Build history of the part. All positions in model axes, mm. Face numbers are marked on the shaded views. A direction names the side the tool comes from. Round coordinates to 2 decimals unless told otherwise and drop trailing zeros. Order: outer loops, then holes, each group sorted by start corner. A loop starts at its lowest first (then second) coordinate and runs counter-clockwise, first axis right, second up. Notation, with made-up numbers: M 78.25,81.5 L 119.25,81.5 A15 cw 119.25,104.5 Z; hole C 34.25,-33.5 d8. An arc over 180 degrees is marked long. One line per item, written item: value. Start each with the question number.
Item 1: Pin check, flat tips, straight feed: pin 1 (5 mm diameter, centred on x = 9, y = -2, fed in from +Z); pin 2 (2.5 mm diameter, centred on x = 0, z = -6.75, fed in from -Y); pin 3 (8 mm diameter, centred on x = -5, z = -13.5, fed in from -Y); pin 4 (10 mm diameter, centred on x = -2, y = -12.5, fed in from +Z). Stop position of each tip, or through.
Item 2: Band-saw the part on B-B, the plane z = 0. Write the cut outline in (x, y), then the cut area to 3 significant figures.
Item 3: Two-plate mould, pull along X, no slides. Class the marked faces 1, 2, 3 and 4: +X half, -X half, draft (parallel to the pull), parting line (faces both ways), or undercut.
Item 4: Probe L1, parallel to X at y = -21.55, z = -17.5; L2, parallel to X at y = 0.25, z = 0; L3, parallel to Y at x = 0, z = 10. List the from-to ranges inside material, lowest first.
Item 5: Tool access for the marked faces 5 and 6: list every direction of +Z, -Z, +X, -X, +Y, -Y with a clear straight run to the whole face (end or side of a thin tool).
Item 6: Band-saw the part on D-D, the plane x = 14.5. Write the cut outline in (y, z).
Item 7: Band-saw the part on C-C, the plane y = -9. Write the cut outline in (x, z), then the cut area to 3 significant figures.
Item 8: Band-saw the part on A-A, the plane x = 0. Write the cut outline in (y, z), then the cut area to 3 significant figures.
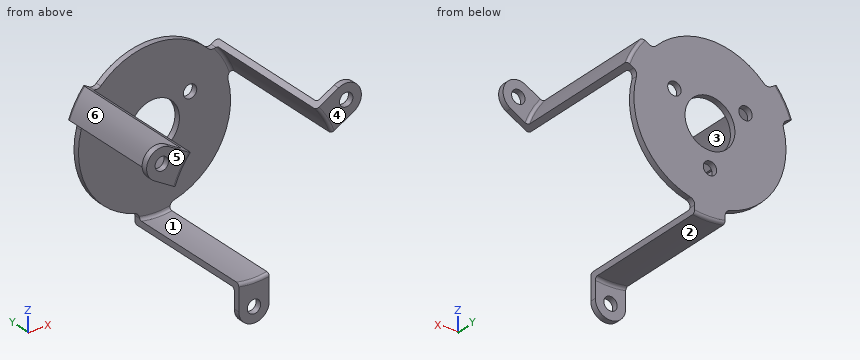
```python
from build123d import *

# Parameters (mm, degrees)
ESBO_O1_R                = 4.1
ESBO_O1_R_2              = 1.099999999999999
ESBO_O1_R_3              = 1.1000000000000312
ESBO_O1_R_4              = 1.1000000000000612
RESSALTO_EXTRUS_O1_DEPTH = 1
RESSALTO_EXTRUS_O2_START = 22.2
RESSALTO_EXTRUS_O2_DEPTH = 22.2
ESBO_O3_R                = 1.1
ESBO_O3_R_2              = 1.100000000000001
ESBO_O3_R_3              = 1.0999999999999976
RESSALTO_EXTRUS_O3_DEPTH = 1
FILETE1_R                = 1
FILETE2_R                = 0.5
FILETE3_R                = 0.5
FILETE4_R                = 0.5
FILETE5_R                = 0.5


with BuildPart() as part:
    # Esboço1 → Ressalto-extrusão1 (new body)
    with BuildSketch(Plane(origin=(0, 0, 0), x_dir=(1, 0, 0), z_dir=(0, 1, 0))):
        with BuildLine():
            Line((-2.5000000000000018, 14.2828568570857), (-2.5000000000000004, 12.24744871391589))
            ThreePointArc((-2.5000000000000004, 12.24744871391589), (-10.825317547305453, 6.250000000000052), (-11.856601717798243, -3.9586608474967395))
            Line((-11.856601717798243, -3.9586608474967395), (-13.619316876853024, -4.976364919081628))
            ThreePointArc((-13.619316876853024, -4.976364919081628), (-12.557368354874425, -7.249999999999881), (-11.119316876853064, -9.306491938003845))
            Line((-11.119316876853064, -9.306491938003845), (-9.356601717798284, -8.288787866418957))
            ThreePointArc((-9.356601717798284, -8.288787866418957), (-8.528e-14, -12.499999999999996), (9.356601717798178, -8.288787866419089))
            Line((9.356601717798178, -8.288787866419089), (11.119316876852942, -9.306491938004001))
            ThreePointArc((11.119316876852942, -9.306491938004001), (12.55736835487433, -7.250000000000061), (13.619316876852963, -4.976364919081819))
            Line((13.619316876852963, -4.976364919081819), (11.856601717798197, -3.958660847496907))
            ThreePointArc((11.856601717798197, -3.958660847496907), (10.8253175473055, 6.249999999999976), (2.499999999999998, 12.24744871391589))
            Line((2.499999999999998, 12.24744871391589), (2.4999999999999982, 14.2828568570857))
            ThreePointArc((2.4999999999999982, 14.2828568570857), (8.9e-16, 14.5), (-2.5000000000000018, 14.2828568570857))
        make_face()
        with Locations(Location((0, 0, 0), (0, 0, 270))):
            Circle(ESBO_O1_R, mode=Mode.SUBTRACT)
        with Locations(Location((0, 6.750000000000001, 0), (0, 0, 270))):
            Circle(ESBO_O1_R_2, mode=Mode.SUBTRACT)
        with Locations(Location((5.845671475544961, -3.374999999999999, 0), (0, 0, 270))):
            Circle(ESBO_O1_R_3, mode=Mode.SUBTRACT)
        with Locations(Location((-5.84567147554496, -3.3750000000000036, 0), (0, 0, 270))):
            Circle(ESBO_O1_R_4, mode=Mode.SUBTRACT)
    extrude(amount=RESSALTO_EXTRUS_O1_DEPTH)

    # Esboço2 → Ressalto-extrusão2 (add)
    with BuildSketch(Plane.XZ.offset(RESSALTO_EXTRUS_O2_START)):
        with BuildLine():
            Line((-11.11931687685307, 9.30649193800384), (-10.239125293076137, 8.798313090171801))
            ThreePointArc((-10.239125293076137, 8.798313090171801), (-11.691342951089984, 6.74999999999989), (-12.739125293076098, 4.4681860712495824))
            Line((-12.739125293076098, 4.4681860712495824), (-13.619316876853024, 4.976364919081628))
            ThreePointArc((-13.619316876853024, 4.976364919081628), (-12.557368354874427, 7.249999999999882), (-11.11931687685307, 9.30649193800384))
        make_face()
        with BuildLine():
            Line((-2.5000000000000018, -14.2828568570857), (-2.5000000000000013, -13.266499161421601))
            ThreePointArc((-2.5000000000000013, -13.266499161421601), (-2.17e-15, -13.500000000000002), (2.499999999999998, -13.266499161421601))
            Line((2.499999999999998, -13.266499161421601), (2.4999999999999982, -14.2828568570857))
            ThreePointArc((2.4999999999999982, -14.2828568570857), (8.9e-16, -14.500000000000002), (-2.5000000000000018, -14.2828568570857))
        make_face()
        with BuildLine():
            Line((13.619316876852963, 4.976364919081819), (12.739125293076041, 4.468186071249766))
            ThreePointArc((12.739125293076041, 4.468186071249766), (11.691342951089894, 6.750000000000058), (10.239125293076022, 8.798313090171948))
            Line((10.239125293076022, 8.798313090171948), (11.119316876852942, 9.306491938004001))
            ThreePointArc((11.119316876852942, 9.306491938004001), (12.557368354874331, 7.250000000000062), (13.619316876852963, 4.976364919081819))
        make_face()
    extrude(amount=-RESSALTO_EXTRUS_O2_DEPTH)

    # Esboço3 → Ressalto-extrusão3 (add)
    # profile 1 of 3: a face of its own
    with BuildSketch(Plane.XZ.offset(22.2)):
        with BuildLine():
            Line((2.4999999999999982, -14.2828568570857), (2.4999999999999982, -17.5))
            ThreePointArc((2.4999999999999982, -17.5), (-1.99e-15, -20), (-2.500000000000002, -17.5))
            Line((-2.500000000000002, -17.5), (-2.5000000000000018, -14.2828568570857))
            ThreePointArc((-2.5000000000000018, -14.2828568570857), (8.9e-16, -14.500000000000002), (2.4999999999999982, -14.2828568570857))
        make_face()
        with Locations(Location((-1.53e-15, -17.5, 0), (0, 0, 270))):
            Circle(ESBO_O3_R, mode=Mode.SUBTRACT)
    # profile 2 of 3: a face of its own
    with BuildSketch(Plane.XZ.offset(22.2)):
        with BuildLine():
            Line((-11.11931687685294, 9.306491938004003), (-13.905444566227628, 10.915063509461165))
            ThreePointArc((-13.905444566227628, 10.915063509461165), (-17.320508075688732, 10.000000000000085), (-16.40544456622765, 6.584936490538983))
            Line((-16.40544456622765, 6.584936490538983), (-13.619316876852961, 4.97636491908182))
            ThreePointArc((-13.619316876852961, 4.97636491908182), (-12.55736835487433, 7.250000000000063), (-11.11931687685294, 9.306491938004003))
        make_face()
        with Locations(Location((-15.15544456622764, 8.750000000000073, 0), (0, 0, 270))):
            Circle(ESBO_O3_R_2, mode=Mode.SUBTRACT)
    # profile 3 of 3: a face of its own
    with BuildSketch(Plane.XZ.offset(22.2)):
        with BuildLine():
            Line((13.619316876853029, 4.976364919081625), (16.40544456622774, 6.58493649053875))
            ThreePointArc((16.40544456622774, 6.58493649053875), (17.320508075688867, 9.999999999999838), (13.905444566227779, 10.915063509460968))
            Line((13.905444566227779, 10.915063509460968), (11.11931687685307, 9.306491938003841))
            ThreePointArc((11.11931687685307, 9.306491938003841), (12.557368354874429, 7.249999999999881), (13.619316876853029, 4.976364919081625))
        make_face()
        with Locations(Location((15.155444566227757, 8.749999999999858, 0), (0, 0, 270))):
            Circle(ESBO_O3_R_3, mode=Mode.SUBTRACT)
    extrude(amount=-RESSALTO_EXTRUS_O3_DEPTH)

    # Filete1
    filete1_edges = [part.edges().sort_by_distance(p)[0] for p in [
        (11.856601717798199, 0.5, 3.9586608474969074),
        (2.4999999999999982, 0.5, -12.24744871391589),
        (-2.5000000000000004, 0.5, -12.24744871391589),
        (-11.856601717798242, 0.5, 3.9586608474967386),
        (9.356601717798178, 0.5, 8.288787866419089),
        (-9.356601717798284, 0.5, 8.288787866418957),
    ]]
    fillet(filete1_edges, radius=FILETE1_R)

    # Filete2
    filete2_edges = [part.edges().sort_by_distance(p)[0] for p in [
        (-12.557368354874423, 1, 7.2499999999998845),
        (12.557368354874328, 1, 7.250000000000058),
        (-2.33e-15, 1, -14.5),
    ]]
    fillet(filete2_edges, radius=FILETE2_R)

    # Filete3
    filete3_edges = [part.edges().sort_by_distance(p)[0] for p in [
        (-1.67e-15, 0, -13.499999999999998),
        (11.691342951089894, 0, 6.750000000000058),
        (-11.691342951089982, 0, 6.749999999999892),
    ]]
    fillet(filete3_edges, radius=FILETE3_R)

    # Filete4
    filete4_edges = [part.edges().sort_by_distance(p)[0] for p in [
        (-12.557368354874328, -21.2, 7.250000000000062),
        (12.55736835487443, -21.2, 7.249999999999882),
        (-1.67e-15, -21.2, -14.500000000000004),
    ]]
    fillet(filete4_edges, radius=FILETE4_R)

    # Filete5
    filete5_edges = [part.edges().sort_by_distance(p)[0] for p in [
        (-1.67e-15, -22.2, -13.499999999999998),
        (-11.691342951089982, -22.2, 6.749999999999892),
        (11.691342951089894, -22.2, 6.750000000000058),
    ]]
    fillet(filete5_edges, radius=FILETE5_R)


solid = part.part
```
Output:
1. pin 1: stops at z = 10
1. pin 2: stops at y = 0
1. pin 3: stops at y = -22.2
1. pin 4: stops at z = -13.27
2. outline: M -12.5,0 L -4.1,0 L -4.1,1 L -12.5,1 Z; M 4.1,0 L 12.5,0 L 12.5,1 L 4.1,1 Z
2. area: 16.8 mm²
3. face 1: undercut
3. face 2: parting line
3. face 3: undercut
3. face 4: draft
4. L1: x = -2.5 to -1.1, 1.1 to 2.5
4. L2: x = -12.5 to -4.1, 4.1 to 12.5
4. L3: y = 0 to 1
5. face 5: +Z, -Z, +X, -X, -Y
5. face 6: +Z, -X, +Y
6. outline: M -22.2,5.48 L -21.2,5.48 L -21.2,7.87 L -22.2,7.87 Z; M -22.2,9.63 L -21.2,9.63 L -21.2,11.16 L -22.2,11.16 Z
7. outline: M -13.62,4.98 L -12.74,4.47 A13.5 cw -10.24,8.8 L -11.12,9.31 A14.5 ccw Z; M -2.5,-14.28 A14.5 ccw 2.5,-14.28 L 2.5,-13.27 A13.5 cw -2.5,-13.27 Z; M 10.24,8.8 A13.5 cw 12.74,4.47 L 13.62,4.98 A14.5 ccw 11.12,9.31 Z
7. area: 15.1 mm²
8. outline: M -22.2,-20 L -21.2,-20 L -21.2,-18.6 L -22.2,-18.6 Z; M -22.2,-16.4 L -21.2,-16.4 L -21.2,-15 A0.5 cw -20.7,-14.5 L 0.5,-14.5 A0.5 ccw 1,-14 L 1,-7.85 L 0,-7.85 L 0,-13 A0.5 cw -0.5,-13.5 L -21.7,-13.5 A0.5 ccw -22.2,-14 Z; M 0,-5.65 L 1,-5.65 L 1,-4.1 L 0,-4.1 Z; M 0,4.1 L 1,4.1 L 1,12.5 L 0,12.5 Z
8. area: 42.1 mm²
